Source: CAD feature listing. Evaluate the final solid. Frame: model axes, mm. Face numbers are marked on the shaded views. A direction names the side the tool comes from. Round coordinates to 2 decimals unless told otherwise and drop trailing zeros. Loops run counter-clockwise (first coordinate to the right, second up) from the corner with the lowest first, then second, coordinate; pieces in that order, holes last.
Item 1: Access query for the marked faces 4 and 5. Directions: +Z, -Z, +X, -X, +Y, -Y. A direction counts if a zero-diameter tool reaches every point of the face in a straight line with its end or side. Return the directions, or none.
Item 2: Ray query, L1, parallel to Y at x = -37.5, z = 3.75; L2, parallel to Y at x = -17.5, z = 2.75; L3, parallel to X at y = -90, z = 3.5. Return the intervals inside material, ascending.
Item 3: Pull-direction query (X, two-part tool) for the marked faces 1, 2 and 3; classes: released by +X, released by -X, zero draft, split by the parting line, or undercut.
Item 4: Section query B-B on x = -42.5. Return loops of the section in (y, z).
Item 5: Section query A-A on z = 5.25. Give the number of separate pieces and of enclosed holes in the cut face, then the cut area to 3 significant figures.
Item 6: Section query C-C on y = -101.5. Return loops of the section in (x, z), then the cut area to 3 significant figures.
Item 7: First-contact query: P1, Ø1.7, axis at x = -47.17, y = -91.47, coming from the +Z side; P2, Ø1, axis at y = -116, z = 6, coming from the -X side; P3, Ø1.5, axis at x = -51.5, z = 4.5, coming from the -Y side. Flat tips, straight axial feed; report the tip coordinate or a pass-through.
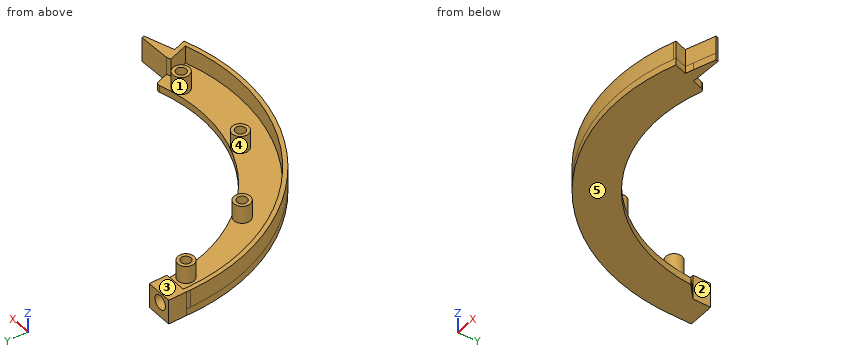
```python
from build123d import *

# Parameters (mm, degrees)
BOSS_EXTRUDE1_DEPTH = 2
BOSS_EXTRUDE2_DEPTH = 5
SKETCH3_R           = 2.3
BOSS_EXTRUDE3_DEPTH = 5
BOSS_EXTRUDE4_DEPTH = 5
SKETCH6_R           = 1.4
CUT_EXTRUDE1_DEPTH  = 5
SKETCH7_R           = 2
CUT_EXTRUDE2_DEPTH  = 8


with BuildPart() as part:
    # Sketch1 → Boss-Extrude1 (new body)
    with BuildSketch(Plane.XY):
        with BuildLine():
            Line((16.887910555, -133.369322594), (14.673679255, -134.127250965))
            Line((14.673679255, -134.127250965), (15.867669408, -137.615404294))
            ThreePointArc((15.867669408, -137.615404294), (-34.007319131, -130.034150274), (-56.342527733, -84.8))
            Line((-56.342527733, -84.8), (-48.940455795, -84.8))
            Line((-48.940455795, -84.8), (-45.096768624, -88.26027792))
            ThreePointArc((-45.096768624, -88.26027792), (-26.483938318, -121.642871269), (11.312186404, -127.325119655))
            ThreePointArc((11.312186404, -127.325119655), (12.064722619, -127.385308804), (12.560733381, -127.954436921))
            Line((12.560733381, -127.954436921), (13.597675192, -130.983785211))
            Line((13.597675192, -130.983785211), (22.508911342, -130.69915726))
            Line((22.508911342, -130.69915726), (22.749464344, -131.362920683))
            Line((22.749464344, -131.362920683), (16.887910555, -133.369322594))
        make_face()
    extrude(amount=BOSS_EXTRUDE1_DEPTH)

    # Sketch2 → Boss-Extrude2 (add)
    with BuildSketch(Plane.XY.offset(2)):
        with BuildLine():
            Line((-56.342527733, -84.8), (-55.142230801, -84.8))
            ThreePointArc((-55.142230801, -84.8), (-55.152352766, -85.399962054), (-55.155726896, -86))
            ThreePointArc((-55.155726896, -86), (-33.342347458, -129.033761126), (14.261826326, -136.880464731))
            Line((14.261826326, -136.880464731), (12.45002618, -131.36047245))
            Line((12.45002618, -131.36047245), (13.597675192, -130.983785211))
            Line((13.597675192, -130.983785211), (15.867669408, -137.615404294))
            ThreePointArc((15.867669408, -137.615404294), (15.540815193, -137.726132378), (15.21326709, -137.834790682))
            ThreePointArc((15.21326709, -137.834790682), (-33.801189066, -130.184178235), (-56.355726896, -86))
            ThreePointArc((-56.355726896, -86), (-56.352427006, -85.399963706), (-56.342527733, -84.8))
        make_face()
    extrude(amount=BOSS_EXTRUDE2_DEPTH)

    # Sketch3 → Boss-Extrude3 (add)
    with BuildSketch(Plane.XY.offset(2)):
        with Locations((7.607262335, -130.722795016)):
            Circle(SKETCH3_R)
        with Locations((-17.271773957, -129.003020951)):
            Circle(SKETCH3_R)
        with Locations((-37.543895432, -114.478381178)):
            Circle(SKETCH3_R)
        with Locations((-47.172740285, -91.473829097)):
            Circle(SKETCH3_R)
        Polygon((14.673679255, -134.127250965), (22.749464344, -131.362920683), (22.508911342, -130.69915726), (13.597675192, -130.983785211), align=None)
    extrude(amount=BOSS_EXTRUDE3_DEPTH)

    # Sketch4 → Boss-Extrude4 (add)
    with BuildSketch(Plane(origin=(0, -84.8, 0), x_dir=(1, 0, 0), z_dir=(0, 1, 0))):
        Polygon((-56.342527733, 0), (-48.940455795, 0), (-48.940455795, -7), (-56.355726896, -7), align=None)
    extrude(amount=BOSS_EXTRUDE4_DEPTH)

    # Sketch6 → Cut-Extrude1 (cut)
    with BuildSketch(Plane.XY.offset(7)):
        with Locations((-47.172740285, -91.473829097)):
            Circle(SKETCH6_R)
        with Locations((-37.543895432, -114.478381178)):
            Circle(SKETCH6_R)
        with Locations((-17.271773957, -129.003020951)):
            Circle(SKETCH6_R)
        with Locations((7.607262335, -130.722795016)):
            Circle(SKETCH6_R)
    extrude(amount=-CUT_EXTRUDE1_DEPTH, mode=Mode.SUBTRACT)

    # Sketch7 → Cut-Extrude2 (cut)
    with BuildSketch(Plane(origin=(0, -79.8, 0), x_dir=(1, 0, 0), z_dir=(0, 1, 0))):
        with Locations(Location((-53.113278602, -4.212750817, 0), (0, 0, 270))):
            Circle(SKETCH7_R)
    extrude(amount=-CUT_EXTRUDE2_DEPTH, mode=Mode.SUBTRACT)


solid = part.part
```
Data:
1. face 4: +Z
1. face 5: -Z, +X, -X, +Y, -Y
2. L1: y = -127.25 to -125.65, -116.78 to -115.88, -113.08 to -112.18
2. L2: y = -138.25 to -136.99, -131.29 to -130.38, -127.62 to -126.71
2. L3: x = -56.21 to -55.01, -48.94 to -45.41
3. face 1: undercut
3. face 2: released by +X
3. face 3: zero draft
4. outline: (-122.33, 0) - (-100.94, 0) - (-100.94, 2) - (-120.5, 2) - (-120.5, 7) - (-122.33, 7) - close
5. separate pieces: 6
5. enclosed holes: 4
5. area: 211 mm2
6. outline: (-54.11, 0) - (-42.29, 0) - (-42.29, 2) - (-52.85, 2) - (-52.85, 7) - (-54.11, 7) - close
6. area: 29.9 mm2
7. P1: stops at z = 2
7. P2: stops at x = -47.69
7. P3: stops at y = -110.09
